from build123d import *

# Parameters (mm, degrees)
SKETCH1_W           = 100
SKETCH1_H           = 8
BOSS_EXTRUDE1_DEPTH = 2.85
CUT_EXTRUDE1_DEPTH  = 51.240645896
SKETCH3_R           = 1.7
CUT_EXTRUDE2_DEPTH  = 51.240645896
SKETCH4_R           = 1.7
CUT_EXTRUDE3_DEPTH  = 51.240645896
CUT_EXTRUDE4_DEPTH  = 51.240645896


with BuildPart() as part:
    # Sketch1 → Boss-Extrude1 (new body)
    with BuildSketch(Plane.XY):
        Rectangle(SKETCH1_W, SKETCH1_H)
    extrude(amount=BOSS_EXTRUDE1_DEPTH)

    # Sketch2 → Cut-Extrude1 (cut, through all)
    with BuildSketch(Plane.XY.offset(2.85)):
        with BuildLine():
            Line((46, -4), (51, -4))
            Line((51, -4), (51, 4))
            Line((51, 4), (46, 4))
            ThreePointArc((46, 4), (50, 0), (46, -4))
        make_face()
    cut_extrude1 = extrude(amount=-CUT_EXTRUDE1_DEPTH, mode=Mode.SUBTRACT)

    # Sketch3 → Cut-Extrude2 (cut, through all)
    with BuildSketch(Plane.XY.offset(2.85)):
        with Locations((46, 0)):
            Circle(SKETCH3_R)
    cut_extrude2 = extrude(amount=-CUT_EXTRUDE2_DEPTH, mode=Mode.SUBTRACT)

    # Mirror1: Cut-Extrude1, Cut-Extrude2 across plane
    add(cut_extrude1.mirror(Plane(origin=(0, 0, 0), x_dir=(0, 0, 1), z_dir=(1, 0, 0))), mode=Mode.SUBTRACT)
    add(cut_extrude2.mirror(Plane(origin=(0, 0, 0), x_dir=(0, 0, 1), z_dir=(1, 0, 0))), mode=Mode.SUBTRACT)

    # Sketch4 → Cut-Extrude3 (cut, through all)
    with BuildSketch(Plane.XY.offset(2.85)):
        with Locations((-19, 0)):
            Circle(SKETCH4_R)
    extrude(amount=-CUT_EXTRUDE3_DEPTH, mode=Mode.SUBTRACT)

    # Sketch5 → Cut-Extrude4 (cut, through all)
    with BuildSketch(Plane.XY.offset(2.85)):
        with BuildLine():
            Line((-19, 4), (-50, 4))
            Line((-50, 4), (-50, -4))
            Line((-50, -4), (-19, -4))
            ThreePointArc((-19, -4), (-23, 0), (-19, 4))
        make_face()
    extrude(amount=-CUT_EXTRUDE4_DEPTH, mode=Mode.SUBTRACT)


solid = part.part
Read the model definition and answer for the solid it produces. Units are mm, in the model's axes. Coordinates: 2 decimals unless noted, no trailing zeros. Order: outer loops, then holes, each group sorted by start corner. A loop starts at its lowest first (then second) coordinate and runs counter-clockwise, first axis right, second up. Notation, with made-up numbers: M 86.25,-29.5 L 101.25,-29.5 A28 ccw 101.25,-2.5 Z; hole C 53,19 d9. An arc over 180 degrees is marked long. Put each result on its own line as item: value. Start each with the question number.
Item 1: Consider probe 1 along Y at (x, z) = (-19, 1.65); probe 2 along X at (y, z) = (1, 1.3); probe 3 along X at (y, z) = (0.25, 1.65). Determine where each line is inside the solid, lowest interval first. Write a range as [from, to].
Item 2: The mould has two halves that part along X. Classify faces 1 (the face through (13, -4, 1)), 2 (the face through (50, 0, 1)), 3 (the face through (-17.43, -0.65, 1.44)): +X half, -X half, draft (parallel to the pull), parting line (faces both ways), or undercut.
Item 3: Given pin 1 Ø2 at (x, y) = (-19, 0) entering from +Z, flat-ended and moving along its own axis, determine where the tip first touches the part or whether it passes through.
Item 4: Section B-B, the plane z = 0.7 is taken. Determine the outline of the cut face in (x, y).
Item 5: Section A-A, the plane y = 0 is taken. Determine the outline of the cut face in (x, z).
Computed:
1. probe 1: y = [-4, -1.7], [1.7, 4]
1. probe 2: x = [-22.87, -20.37], [-17.63, 44.63], [47.37, 49.87]
1. probe 3: x = [-22.99, -20.68], [-17.32, 44.32], [47.68, 49.99]
2. face 1: draft
2. face 2: +X half
2. face 3: undercut
3. pin 1: passes through
4. outline: M -19,-4 L 46,-4 A4 ccw 46,4 L -19,4 A4 ccw Z; hole C -19,0 d3.4; hole C 46,0 d3.4
5. outline: M -23,0 L -20.7,0 L -20.7,2.85 L -23,2.85 Z; M -17.3,0 L 44.3,0 L 44.3,2.85 L -17.3,2.85 Z; M 47.7,0 L 50,0 L 50,2.85 L 47.7,2.85 Z
